Part model, mm, in its own coordinate system. Face numbers are marked on the shaded views. A direction names the side the tool comes from. Give positions to 0.01 mm unless a question says otherwise; leave off trailing zeros. Order: outer loops, then holes, each group sorted by start corner. A loop starts at its lowest first (then second) coordinate and runs counter-clockwise, first axis right, second up. Notation, with made-up numbers: M 5.25,3.25 L 59.25,3.25 A17 cw 59.25,19.25 Z; hole C 69,8.25 d11. An arc over 180 degrees is marked long. Write each question's results on one line, items separated by ' | '. Start each with the question number.
from build123d import *

# Parameters (mm, degrees)
SKETCH1_R           = 1.5
BOSS_EXTRUDE1_DEPTH = 15
SKETCH2_R           = 2.75
BOSS_EXTRUDE2_DEPTH = 3
CUT_EXTRUDE1_DEPTH  = 2
CHAMFER1_SIZE       = 0.1


with BuildPart() as part:
    # Sketch1 → Boss-Extrude1 (new body)
    with BuildSketch(Plane.XY):
        Circle(SKETCH1_R)
    extrude(amount=-BOSS_EXTRUDE1_DEPTH)

    # Sketch2 → Boss-Extrude2 (add)
    with BuildSketch(Plane.XY):
        Circle(SKETCH2_R)
    extrude(amount=BOSS_EXTRUDE2_DEPTH)

    # Sketch3 → Cut-Revolve1 (revolve, cut)
    with BuildSketch(Plane(origin=(0, 0, 0), x_dir=(0, 0, -1), z_dir=(1, 0, 0)), mode=Mode.PRIVATE) as cut_revolve1_sk:
        with BuildLine():
            Line((-3, 2.6), (-3, 3.1))
            Line((-3, 3.1), (0, 3.1))
            Line((0, 3.1), (0, 2.6))
            Line((0, 2.6), (-0.5, 2.6))
            ThreePointArc((-0.5, 2.6), (-1.75, 2.7), (-3, 2.6))
        make_face()
    revolve(cut_revolve1_sk.sketch.rotate(Axis((0, 0, 3), (0, 0, 1)), 90), axis=Axis((0, 0, 3), (0, 0, 1)), mode=Mode.SUBTRACT)

    # Sketch4 → Cut-Extrude1 (cut)
    with BuildSketch(Plane.XY.offset(3)):
        Polygon((1.732050808, 0), (0.866025404, 1.5), (-0.866025404, 1.5), (-1.732050808, 0), (-0.866025404, -1.5), (0.866025404, -1.5), align=None)
    extrude(amount=-CUT_EXTRUDE1_DEPTH, mode=Mode.SUBTRACT)

    # Chamfer1
    chamfer1_edges = [part.edges().sort_by_distance(p)[0] for p in [
        (1.299038106, -0.75, 3),
        (1.299038106, 0.75, 3),
        (0, 1.5, 3),
        (-1.299038106, 0.75, 3),
        (-1.299038106, -0.75, 3),
        (0, -1.5, 3),
    ]]
    chamfer(chamfer1_edges, length=CHAMFER1_SIZE)


solid = part.part
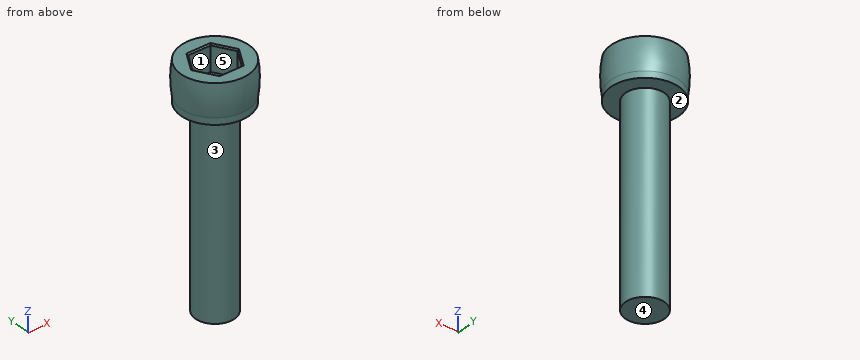
(1) Pull direction Y, two halves, no side cores. Call the marked faces 1, 2 and 3: +Y half, -Y half, draft (parallel to the pull), parting line (faces both ways), or undercut.
(2) Tool access for the marked faces 4 and 5: list every direction of +Z, -Z, +X, -X, +Y, -Y with a clear straight run to the whole face (end or side of a thin tool).
(3) Drop flat-ended pins along their axis: P1, Ø0.5, axis at x = 0, z = 2, coming from the -Y side; P2, Ø1, axis at x = 0, z = -3, coming from the -Y side; P3, Ø0.9, axis at x = 0.5, y = 0, coming from the +Z side; P4, Ø1, axis at x = -1, z = -2, coming from the -Y side. Give the stop position or say it passes through.
(4) Saw through at A-A on z = -5.5. Give the cut face in (x, y), plus the area to 3 significant figures.
(5) Probe L1, parallel to Z at x = 1.25, y = -0.5; L2, parallel to Z at x = 0.05, y = -1.7; L3, parallel to Y at x = 0, z = -4.5. List the from-to ranges inside material, lowest first.
Taken from the geometry:
1) face 1: undercut | face 2: draft | face 3: parting line
2) face 4: -Z, +X, -X, +Y, -Y | face 5: +Z
3) P1: stops at y = -2.7 | P2: stops at y = -1.5 | P3: stops at z = 1 | P4: stops at y = -1.41
4) outline: C 0,0 d3 | area: 7.07 mm²
5) L1: z = -15 to 1 | L2: z = 0 to 3 | L3: y = -1.5 to 1.5
